Input: part model. Units: mm. Frame: model coordinates. Face numbers are marked on the shaded views. A direction names the side the tool comes from. Give positions to 0.01 mm unless a question says otherwise; leave off trailing zeros. Write each loop counter-clockwise with the first axis right and the second up, starting at its lowest first coordinate (ties: lowest second). Pieces come first, ordered by that corner, then holes. Notation, with made-up numbers: (48.25, 55) - (93.25, 55) arc R10 cw to (93.25, 72) - close; hole circle Ø11 at (-35, 60). An arc over 180 degrees is marked (long way). Answer as CSV lines item,"result".
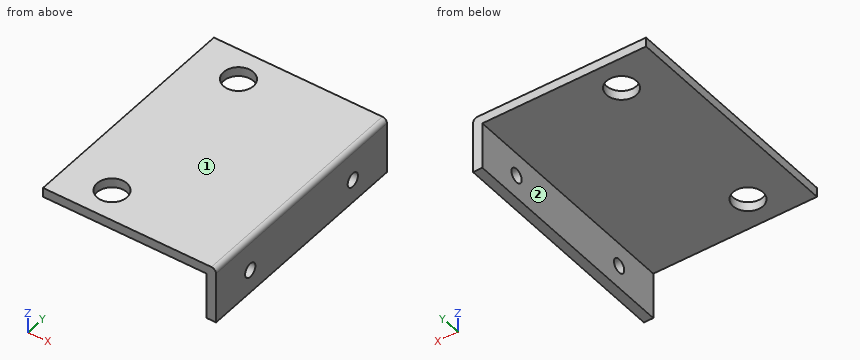
```python
from build123d import *

# Parameters (mm, degrees)
BOSS_EXTRUDE1_DEPTH = 50
FILLET2_R           = 1
SKETCH4_R           = 1.5
CUT_EXTRUDE1_DEPTH  = 64.348243859
SKETCH5_R           = 3.2
CUT_EXTRUDE2_DEPTH  = 64.348243859


with BuildPart() as part:
    # Sketch3 → Boss-Extrude1 (new body)
    with BuildSketch(Plane(origin=(0, 0, 0), x_dir=(1, 0, 0), z_dir=(0, 1, 0))):
        Polygon((0, 0), (37, 0), (37, 12), (35, 12), (35, 2), (0, 2), align=None)
    extrude(amount=BOSS_EXTRUDE1_DEPTH)

    # Fillet2
    fillet2_edges = [part.edges().sort_by_distance(p)[0] for p in [
        (37, 25, 0),
    ]]
    fillet(fillet2_edges, radius=FILLET2_R)

    # Sketch4 → Cut-Extrude1 (cut, through all)
    with BuildSketch(Plane(origin=(37, 0, 0), x_dir=(0, 0, -1), z_dir=(1, 0, 0))):
        with Locations((7, 40)):
            Circle(SKETCH4_R)
        with Locations((7, 10)):
            Circle(SKETCH4_R)
    extrude(amount=-CUT_EXTRUDE1_DEPTH, mode=Mode.SUBTRACT)

    # Sketch5 → Cut-Extrude2 (cut, through all)
    with BuildSketch(Plane.XY):
        with Locations((10, 43.5)):
            Circle(SKETCH5_R)
        with Locations((10, 6.5)):
            Circle(SKETCH5_R)
    extrude(amount=-CUT_EXTRUDE2_DEPTH, mode=Mode.SUBTRACT)


solid = part.part
```
Item 1: Cut plane C-C on x = 10. Return the cut outline in (y, z), plus the area to 3 significant figures.
The answers:
outline,"(0, -2) - (3.3, -2) - (3.3, 0) - (0, 0) - close; (9.7, -2) - (40.3, -2) - (40.3, 0) - (9.7, 0) - close; (46.7, -2) - (50, -2) - (50, 0) - (46.7, 0) - close"
area,"74.4 mm²"
Item 2: Reachability of the marked faces 1 and 2 from +Z, -Z, +X, -X, +Y, -Y: full face, straight path, thin tool, end or side. Return the list, or none.
The answers:
face 1,"+Z, +X, -X, +Y, -Y"
face 2,"-Z, -X, +Y, -Y"
Item 3: Ray query, line 1 (Y direction, x = 35.55, z = -7); line 2 (Y direction, x = 10, z = -1.4); line 3 (Z direction, x = 26, y = 6). Return the intervals inside material, ascending. Write a range as from..to.
The answers:
line 1,"0..8.5, 11.5..38.5, 41.5..50"
line 2,"0..3.3, 9.7..40.3, 46.7..50"
line 3,"-2..0"
Item 4: Cut plane A-A on y = 6.5. Return the cut outline in (x, z), plus the area to 3 significant figures.
The answers:
outline,"(0, -2) - (6.8, -2) - (6.8, 0) - (0, 0) - close; (13.2, -2) - (35, -2) - (35, -12) - (37, -12) - (37, -1) arc R1 ccw to (36, 0) - (13.2, 0) - close"
area,"81.0 mm²"
Item 5: Cut plane B-B on z = -7. Return the cut outline in (x, y), plus the area to 3 significant figures.
The answers:
outline,"(35, 0) - (37, 0) - (37, 8.5) - (35, 8.5) - close; (35, 11.5) - (37, 11.5) - (37, 38.5) - (35, 38.5) - close; (35, 41.5) - (37, 41.5) - (37, 50) - (35, 50) - close"
area,"88.0 mm²"
Item 6: Contact query for flat-ended pins moving along their axis: pin 1 (17.5 mm diameter, centred on x = 20.5, y = 17, fed in from -Z); pin 2 (3.5 mm diameter, centred on y = 40, z = -7, fed in from -X); pin 3 (5 mm diameter, centred on x = 10, y = 43.5, fed in from -Z). Output: stop coordinate, or through.
The answers:
pin 1,"z = -2"
pin 2,"x = 35"
pin 3,"through"
Item 7: Cut plane D-D on y = 34.5. Return the cut outline in (x, z), plus the area to 3 significant figures.
The answers:
outline,"(0, -2) - (35, -2) - (35, -12) - (37, -12) - (37, -1) arc R1 ccw to (36, 0) - (0, 0) - close"
area,"93.8 mm²"
